Here's how the part is built. I have some questions about the finished solid (model axes, mm). A direction names the side the tool comes from. Round coordinates to 2 decimals unless told otherwise and drop trailing zeros. Order: outer loops, then holes, each group sorted by start corner. A loop starts at its lowest first (then second) coordinate and runs counter-clockwise, first axis right, second up. Notation, with made-up numbers: (-27.75, -14.75) -> (-3.75, -14.75) arc R23 cw to (-3.75, 12.25) -> close; hole circle Ø8 at (77, -7). An arc over 180 degrees is marked (long way). One line per item, written item: value.
```python
from build123d import *

# Parameters (mm, degrees)
SKETCH_2_W                = 32
SKETCH_2_H                = 30
EXTRUDE_1_DEPTH           = 11
HOLE_WIZARD_1_D           = 3.5
HOLE_WIZARD_1_CBORE_D     = 6
HOLE_WIZARD_1_CBORE_DEPTH = 20
SKETCH_11_W               = 19.2
SKETCH_11_H               = 12.5
CUT_EXTRUDE_1_DEPTH       = 17
HOLE_WIZARD_M6_1_D        = 5
CHAMFER_1_SIZE            = 1
FILLET_1_R                = 3


# Read off the part's stored shape, not the designer's step: 1/8 Rc 螺纹孔1
with BuildPart() as part:
    # 草图2 → 凸台-拉伸1 (new, symmetric)
    with BuildSketch(Plane.XY):
        Rectangle(SKETCH_2_W, SKETCH_2_H)
    extrude(amount=EXTRUDE_1_DEPTH, both=True)

    # 打孔尺寸根据内六角圆柱头螺钉的类型1 (through all)
    with Locations(Plane.XY.offset(11)):
        with Locations((-0.2, 7.5), (-0.2, -7.5), (9, -7.5)):
            CounterBoreHole(HOLE_WIZARD_1_D / 2, HOLE_WIZARD_1_CBORE_D / 2, HOLE_WIZARD_1_CBORE_DEPTH)

    # 草图11 → 切除-拉伸1 (cut)
    with BuildSketch(Plane.XY.offset(11)):
        with Locations((6.4, -8.75)):
            Rectangle(SKETCH_11_W, SKETCH_11_H)
        with Locations((6.4, 8.75)):
            Rectangle(SKETCH_11_W, SKETCH_11_H)
    extrude(amount=-CUT_EXTRUDE_1_DEPTH, mode=Mode.SUBTRACT)

    # M6 螺纹孔1 (through all)
    with Locations(Plane(origin=(0, -2.5, 0), x_dir=(-1, 0, 0), z_dir=(0, -1, 0))):
        with Locations((-9, -2.5)):
            Hole(HOLE_WIZARD_M6_1_D / 2)

    # 草图9 → 1/8 Rc 螺纹孔2 (revolve, cut)
    with BuildSketch(Plane(origin=(-9.6, -15, 3), x_dir=(0, 0, -1), z_dir=(1, 0, 0))):
        Polygon((0, 0), (0, 22.373399445), (3.95, 20), (3.95, 10), (4.632996789, 10), (4.945163, 0), align=None)
    revolve(axis=Axis((-9.6, -21.35, 3), (0, 1, 0)), mode=Mode.SUBTRACT)

    # 1/8 Rc 螺纹孔1 outline → 1/8 Rc 螺纹孔1 (revolve, cut)
    with BuildSketch(Plane(origin=(-9.6, 0, 3), x_dir=(1, 0, 0), z_dir=(0, 0, 1))):
        Polygon((4.632997031, 7), (4.88273, 15), (0, 15), (0, 7.373399445), (3.95, 5), (3.95, 7), align=None)
    revolve(axis=Axis((-9.6, 0, 3), (0, 1, 0)), mode=Mode.SUBTRACT)

    # 倒角1
    chamfer_1_edges = [part.edges().sort_by_distance(p)[0] for p in [
        (-9.6, -15, 11),
        (16, 0, 11),
        (16, -15, -8.5),
        (-9.6, 15, 11),
        (16, 15, -8.5),
    ]]
    chamfer(chamfer_1_edges, length=CHAMFER_1_SIZE)

    # 圆角1
    fillet_1_edges = [part.edges().sort_by_distance(p)[0] for p in [
        (-3.2, -2.5, 2.5),
        (-3.2, 2.5, 2.5),
    ]]
    fillet(fillet_1_edges, radius=FILLET_1_R)


solid = part.part
```
Q1. Which directions (+Z, -Z, +X, -X, +Y, -Y) give clear straight access to the entire face, cutting with the end or side of a thin tool? Please do faces 4 (the face through (-11, -5, 7)), 5 (the face through (-3.2, 10, 3)), 6 (the face through (-2.34, -3.4, 2.38)), 7 (the face through (-5.06, 11.06, 1.57)), 8 (the face through (10.61, -4.97, -7.48)).
Answers:
face 4: -Y
face 5: +Z, +X, +Y
face 6: +Z, +X, -Y
face 7: +Y
face 8: +Z
Q2. I want a section at D-D on z = -5.5. Write out the boundary of the cut face in (x, y), then the cut area to 3 significant figures.
Answers:
outline: (-16, -15) -> (-3.2, -15) -> (-3.2, -5.5) arc R3 cw to (-0.2, -2.5) -> (16, -2.5) -> (16, 2.5) -> (-0.2, 2.5) arc R3 cw to (-3.2, 5.5) -> (-3.2, 15) -> (-16, 15) -> close
area: 484 mm2
Q3. For P1, Ø5.5, axis at x = -0.2, y = -7.5, coming from the -Z side; P2, Ø8, axis at x = 4, z = 4, coming from the +Y side; P3, Ø10, axis at x = 10.5, y = 11.5, coming from the +Z side; P4, Ø6, axis at y = -11.5, z = 5, coming from the +X side, each with a flat end and sliding along its axis, tell me the tip position at first contact or that it passes through.
Answers:
P1: z = -11
P2: y = 2.5
P3: z = -6
P4: x = -3.2
Q4. I want a section at C-C on x = -9.6. Write out the boundary of the cut face in (y, z).
Answers:
outline: (-15, -11) -> (15, -11) -> (15, -1.88) -> (7, -1.63) -> (7, -0.95) -> (-5, -0.95) -> (-5, -1.63) -> (-15, -1.95) -> close; (-15, 7.95) -> (-5, 7.63) -> (-5, 6.95) -> (7, 6.95) -> (7, 7.63) -> (15, 7.88) -> (15, 10) -> (14, 11) -> (-14, 11) -> (-15, 10) -> close
Q5. I want a section at B-B on y = 6.5. Write out the boundary of the cut face in (x, z), then the cut area to 3 significant figures.
Answers:
outline: (-16, -11) -> (-1.64, -11) -> (-1.64, -9) -> (-3.03, -9) -> (-3.03, -6) -> (-3.2, -6) -> (-3.2, 11) -> (-16, 11) -> close; (1.24, -11) -> (16, -11) -> (16, -6) -> (2.63, -6) -> (2.63, -9) -> (1.24, -9) -> close; hole circle Ø7.9 at (-9.6, 3)
area: 306 mm2
Q6. I need wall thicknesses on line 1 along Y through (x, z) = (-0.2, -7.8); line 2 along X through (y, z) = (7.5, -7.55); line 3 along Y through (x, z) = (9, -6.8). Which ranges of each line are inside material? Lowest first, please.
Answers:
line 1: -15 to -10.5, -4.5 to 4.5, 10.5 to 15
line 2: -16 to -3.2, 2.8 to 16
line 3: -15 to -10.5, -4.5 to 15
Q7. If we mould it in two halves opening along X, with no side actions, what happens to faces 1 (the face through (16, 0, -4)), 2 (the face through (0, 0, -11)), 3 (the face through (2.66, 8.4, -7.48))? For each: pulls with the +X half, pulls with the -X half, needs draft (parallel to the pull), parting line crosses it, or undercut.
Answers:
face 1: pulls with the +X half
face 2: needs draft
face 3: undercut
Q8. I want a section at A-A on x = 9. Write out the boundary of the cut face in (y, z), then the cut area to 3 significant figures.
Answers:
outline: (-15, -11) -> (-9.25, -11) -> (-9.25, -9) -> (-10.5, -9) -> (-10.5, -6) -> (-15, -6) -> close; (-5.75, -11) -> (15, -11) -> (15, -6) -> (2.5, -6) -> (2.5, 0) -> (-2.5, 0) -> (-2.5, -6) -> (-4.5, -6) -> (-4.5, -9) -> (-5.75, -9) -> close; (-2.5, 5) -> (2.5, 5) -> (2.5, 11) -> (-2.5, 11) -> close
area: 185 mm2
